```python
from build123d import *

# Parameters (mm, degrees)
SKETCH1_W           = 55
SKETCH1_H           = 39.2
BOSS_EXTRUDE1_DEPTH = 30
SKETCH2_R           = 16.818308595
CUT_EXTRUDE1_DEPTH  = 46.170897711
SKETCH3_R           = 5.5
CUT_EXTRUDE2_DEPTH  = 6.3
SKETCH5_R           = 3.25
CUT_EXTRUDE3_DEPTH  = 57.505663433


with BuildPart() as part:
    # Sketch1 → Boss-Extrude1 (new body)
    with BuildSketch(Plane(origin=(0, 0, 0), x_dir=(1, 0, 0), z_dir=(0, 1, 0))):
        Rectangle(SKETCH1_W, SKETCH1_H)
    extrude(amount=BOSS_EXTRUDE1_DEPTH)

    # Sketch2 → Cut-Extrude1 (cut, through all)
    with BuildSketch(Plane.XZ):
        with Locations(Location((0, 2.1, 0), (0, 0, 270))):
            Circle(SKETCH2_R)
    extrude(amount=-CUT_EXTRUDE1_DEPTH, mode=Mode.SUBTRACT)

    # Sketch3 → Cut-Extrude2 (cut)
    with BuildSketch(Plane.XY.offset(19.6)):
        with Locations((-21, 23.5)):
            Circle(SKETCH3_R)
        with Locations((-21, 6.5)):
            Circle(SKETCH3_R)
        with Locations(Location((21, 6.5, 0), (0, 0, 180))):
            Circle(SKETCH3_R)
        with Locations(Location((21, 23.5, 0), (0, 0, 180))):
            Circle(SKETCH3_R)
    extrude(amount=-CUT_EXTRUDE2_DEPTH, mode=Mode.SUBTRACT)

    # Sketch5 → Cut-Extrude3 (cut, through all)
    with BuildSketch(Plane.XY.offset(19.6)):
        with Locations((-21, 6.5)):
            Circle(SKETCH5_R)
        with Locations((-21, 23.5)):
            Circle(SKETCH5_R)
        with Locations(Location((21, 23.5, 0), (0, 0, 180))):
            Circle(SKETCH5_R)
        with Locations(Location((21, 6.5, 0), (0, 0, 180))):
            Circle(SKETCH5_R)
    extrude(amount=-CUT_EXTRUDE3_DEPTH, mode=Mode.SUBTRACT)


solid = part.part
```
Can you work these out from the model? Positions are in its coordinate system, mm. A direction names the side the tool comes from. Coordinates: 2 decimals unless noted, no trailing zeros. Order: outer loops, then holes, each group sorted by start corner. A loop starts at its lowest first (then second) coordinate and runs counter-clockwise, first axis right, second up.
1. I need wall thicknesses on line 1 (Y direction, x = -21, z = 0); line 2 (Y direction, x = 21, z = 16.75); line 3 (X direction, y = 8.75, z = -17). Which ranges of each line are inside material? Lowest first, please.
2. If we section it at B-B (z = 2.1): Please give me the cut outline in (x, y), then the cut area to 3 significant figures.
3. Thinking about a two-plate mould opening in X: for faces 1 (the face through (-27.5, 15, 0)), 2 (the face through (-10.23, 14.79, 15.45)), 3 (the face through (0, 0, -18)), which applies, +X half, -X half, draft (parallel to the pull), parting line (faces both ways), or undercut?
4. If we section it at C-C (x = 13): Please give me the cut outline in (y, z), then the cut area to 3 significant figures.
5. For faces 4 (the face through (-21, 3, 13.3)), 5 (the face through (0, 15, -19.6)), which set-ups out of +Z, -Z, +X, -X, +Y, -Y let a thin tool reach every point of the face, with its end or its side?
6. I'm going to push flat-ended pins straight in: pin 1 (1 mm diameter, centred on x = 20.5, y = 24.5, fed in from -Z); pin 2 (10.5 mm diameter, centred on x = -21, y = 23.5, fed in from +Z). Where does each tip first touch, or does it pass through?
7. If we section it at D-D (y = 16.5): Please give me the cut outline in (x, z).
8. If we section it at A-A (y = 6.5): Please give me the cut outline in (x, z).
Entries:
1. line 1: y = 0 to 3.25, 9.75 to 20.25, 26.75 to 30
1. line 2: y = 0 to 1, 12 to 18, 29 to 30
1. line 3: x = -27.5 to -23.35, -18.65 to 18.65, 23.35 to 27.5
2. outline: (-27.5, 0) - (-16.82, 0) - (-16.82, 30) - (-27.5, 30) - close; (16.82, 0) - (27.5, 0) - (27.5, 30) - (16.82, 30) - close; hole circle Ø6.5 at (-21, 6.5); hole circle Ø6.5 at (-21, 23.5); hole circle Ø6.5 at (21, 6.5); hole circle Ø6.5 at (21, 23.5)
2. area: 508 mm2
3. face 1: -X half
3. face 2: undercut
3. face 3: draft
4. outline: (0, -19.6) - (30, -19.6) - (30, -8.57) - (0, -8.57) - close; (0, 12.77) - (30, 12.77) - (30, 19.6) - (0, 19.6) - close
4. area: 536 mm2
5. face 4: +Z
5. face 5: -Z, +X, -X, +Y, -Y
6. pin 1: passes through
6. pin 2: stops at z = 13.3
7. outline: (-27.5, -19.6) - (27.5, -19.6) - (27.5, 19.6) - (-27.5, 19.6) - close; hole circle Ø33.64 at (0, 2.1)
8. outline: (-27.5, -19.6) - (-24.25, -19.6) - (-24.25, 13.3) - (-26.5, 13.3) - (-26.5, 19.6) - (-27.5, 19.6) - close; (-17.75, -19.6) - (17.75, -19.6) - (17.75, 13.3) - (15.5, 13.3) - (15.5, 19.6) - (-15.5, 19.6) - (-15.5, 13.3) - (-17.75, 13.3) - close; (24.25, -19.6) - (27.5, -19.6) - (27.5, 19.6) - (26.5, 19.6) - (26.5, 13.3) - (24.25, 13.3) - close; hole circle Ø33.64 at (0, 2.1)
